The model under review builds one solid part; all positions refer to its coordinate system, in mm. Face numbers are marked on the shaded views. A direction names the side the tool comes from. Round coordinates to 2 decimals unless told otherwise and drop trailing zeros. Write each loop counter-clockwise with the first axis right and the second up, starting at its lowest first coordinate (ties: lowest second). Pieces come first, ordered by that corner, then holes. Notation, with made-up numbers: (76.25, 76.25) -> (110.25, 76.25) arc R31 cw to (110.25, 115.25) -> close; hole circle Ø7 at (5.5, 63). An arc over 180 degrees is marked (long way). Return JSON: item names as keys, results as strings. Group by question number.
1. Clearance check with flat-ended pins moving along their axes: P1, Ø16, axis at x = 1, y = 35, coming from the -Z side; P2, Ø12, axis at x = -5, z = 41.5, coming from the +Y side. State where each tip first meets the part, or that it passes through.
2. Take a section at D-D, the plane y = 30.5. Write out the cut boundary in (x, z), then the cut area to 3 significant figures.
3. Take a section at B-B, the plane z = 0. Write out the cut boundary in (x, y) (3 decimals), then the cut area to 3 significant figures.
4. Tool access review of the marked faces 1 and 2: name each direction out of +Z, -Z, +X, -X, +Y, -Y from which nothing blocks a thin tool from reaching the whole face with its end or side.
5. Take a section at C-C, the plane z = 113.5. Write out the cut boundary in (x, y).
6. For line 1 along X through (y, z) = (71, 146); line 2 along X through (y, z) = (6, 0) (3 decimals); line 3 along Z through (x, y) = (0, 0.9), list the stretches that pass through material, from the lowest coordinate up. Write a range as from..to.
7. Take a section at A-A, the plane x = 0. Write out the cut boundary in (y, z) (3 decimals).
Autodesk Inventor part; units mm, degrees
ref_plane "YZ Plane" through (0, 0, 0) normal (1, 0, 0) x (0, 1, 0)
ref_plane "XZ Plane" through (0, 0, 0) normal (0, 1, 0) x (-1, 0, 0)
ref_plane "XY Plane" through (0, 0, 0) normal (0, 0, 1) x (1, 0, 0)
sketch "스케치1" plane through (0, 0, 0) normal (0, 1, 0) x (-1, 0, 0)
  circle A0 centre (0, 0) radius 16.025
  circle A1 centre (0, 0) radius 28
  dimension "d0" = 32.05
  dimension "d1" = 56
extrude "돌출1" add sketch "스케치1" along normal blind 9
sketch "스케치2" plane through (0, 0, 0) normal (0, -1, 0) x (1, 0, 0)
  circle A0 centre (0, 0) radius 13
  circle A1 centre (0, 0) radius 16.025
  dimension "d4" = 26
extrude "돌출2" add sketch "스케치2" against normal blind 2
sketch "스케치3" plane through (0, 0, 0) normal (0, -1, 0) x (1, 0, 0)
  circle A0 centre (0, 0) radius 28
  line L0 (-10, 26.1534) -> (10, 26.1534)
  line L1 (10, 26.1534) -> (10, 150)
  line L2 (10, 150) -> (-10, 150)
  line L3 (-10, 150) -> (-10, 26.1534)
  dimension "d7" = 20
  dimension "d8" = 10
  dimension "d15" = 150
extrude "돌출3" add sketch "스케치3" against normal up to surface (9 mm away) contours A0 L3 L2 L1
sketch "스케치4" plane through (0, 9, 0) normal (0, 1, 0) x (1, 0, 0)
  line L0 (10, -150) -> (-10, -150)
  line L1 (10, -150) -> (-10, -150)
  line L2 (-10, -150) -> (-10, -142)
  line L3 (-10, -142) -> (10, -142)
  line L4 (10, -142) -> (10, -150)
  point P0 (0, 0)
  dimension "d12" = 8
extrude "돌출4" add sketch "스케치4" along normal blind 69
fillet "모깎기1" radius 6 2 edges at (10, 4.5, 26.1534) (-10, 4.5, 26.1534)
sketch "스케치5" plane through (0, 78, 0) normal (0, 1, 0) x (1, 0, 0)
  circle A0 centre (-5, -146) radius 1.55
  circle A1 centre (5, -146) radius 1.55
  point P0 (0, 0)
hole "구멍1" at (-5, 78, 146) at (5, 78, 146) direction (0, -1, 0) diameter 3.88 depth 10 tip angle 118 countersink diameter 4.34 countersink angle 7
fillet "모깎기2" radius 6 1 edges at (0, 9, 142)
properties part number "test_arm"
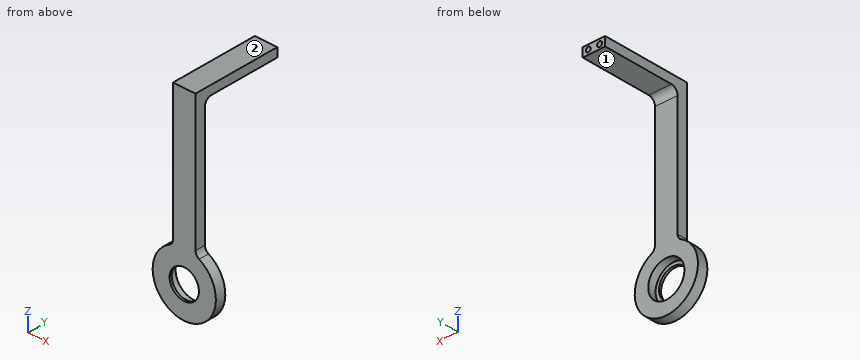
Output:
{
 "1": {"P1": "stops at z = 142", "P2": "stops at y = 9"},
 "2": {"outline": "(-10, 142) -> (10, 142) -> (10, 150) -> (-10, 150) -> close", "area": "160 mm^2"},
 "3": {"outline": "(-28, 0) -> (-13, 0) -> (-13, 2) -> (-16.025, 2) -> (-16.025, 9) -> (-28, 9) -> close; (13, 0) -> (28, 0) -> (28, 9) -> (16.025, 9) -> (16.025, 2) -> (13, 2) -> close", "area": "228 mm^2"},
 "4": {"face 1": "-Z, +X, -X, +Y", "face 2": "+Z, +X, -X, +Y, -Y"},
 "5": {"outline": "(-10, 0) -> (10, 0) -> (10, 9) -> (-10, 9) -> close"},
 "6": {"line 1": "x = -10..-6.94, -3.06..3.06, 6.94..10", "line 2": "x = -28..-16.025, 16.025..28", "line 3": "z = -28..-13, 13..150"},
 "7": {"outline": "(0, -28) -> (9, -28) -> (9, -16.025) -> (2, -16.025) -> (2, -13) -> (0, -13) -> close; (0, 13) -> (2, 13) -> (2, 16.025) -> (9, 16.025) -> (9, 136) arc R6 cw to (15, 142) -> (78, 142) -> (78, 150) -> (0, 150) -> close"}
}
